Print and shaded views of the part. All mm, measured from the part's lowest x, y and z. Round coordinates to 2 decimals unless told otherwise and drop trailing zeros. Write each loop counter-clockwise with the first axis right and the second up, starting at its lowest first coordinate (ties: lowest second). Pieces come first, ordered by that corner, then holes. Notation, with made-up numbers: M 63,87.5 L 97,87.5 A7 ccw 97,92.5 Z; hole C 8.25,7 d6. An arc over 180 degrees is marked long. Write item = value, one per line.
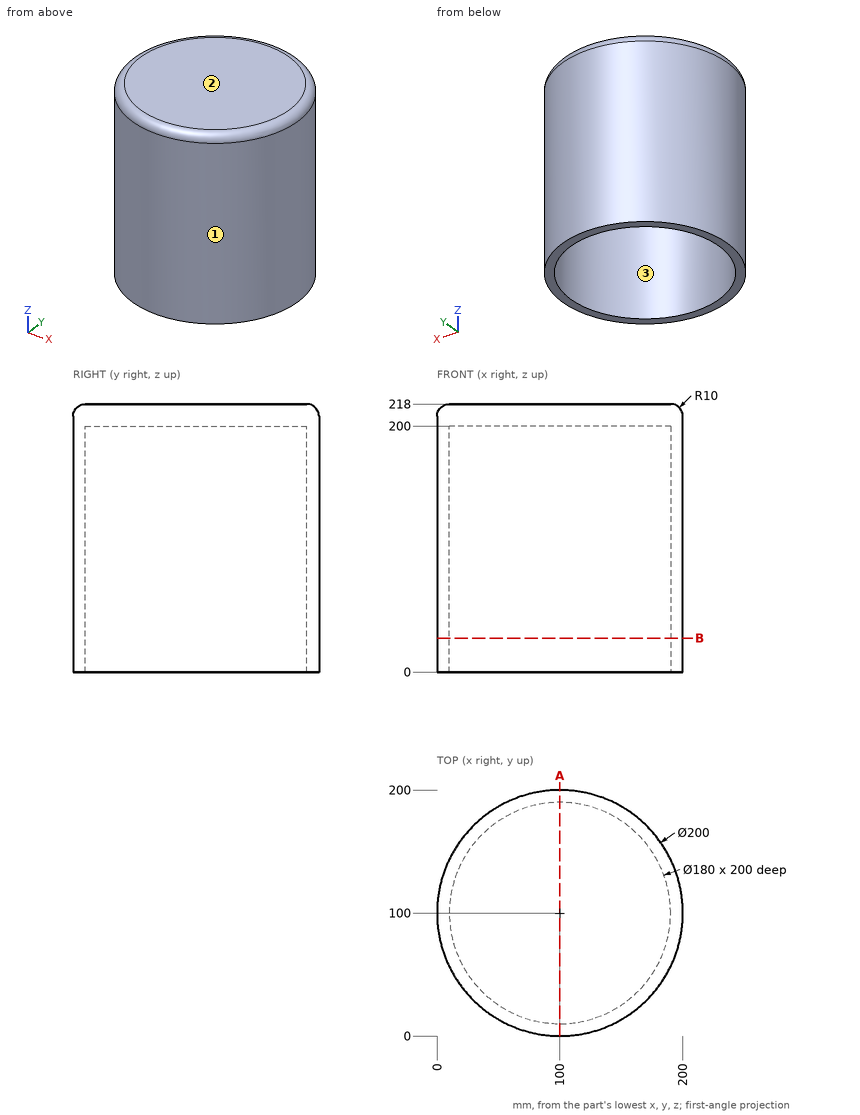
1. Mould opens along X. For the marked faces 1, 2 and 3 say: pulls with the +X half, pulls with the -X half, needs draft (parallel to the pull), parting line crosses it, or undercut.
Responses:
face_1 = parting line crosses it
face_2 = needs draft
face_3 = undercut
2. Band-saw the part on A-A (x = 100). List the corners of the cut face in (y, z).
Responses:
outline = M 0,0 L 10,0 L 10,200 L 190,200 L 190,0 L 200,0 L 200,208 A10 ccw 190,218 L 10,218 A10 ccw 0,208 Z
3. Flat gauge pins, fed straight in: pin 1 (2 mm diameter, centred on x = 126, y = 101.5, fed in from -Z); pin 2 (5 mm diameter, centred on x = 179.5, z = 79, fed in from +Y); pin 3 (8 mm diameter, centred on x = 67.5, z = 156, fed in from +Y). Where does each tip first touch, or does it go through?
Responses:
pin_1 = 200
pin_2 = 163.8
pin_3 = 195.85
4. Band-saw the part on B-B (z = 27.5). List the corners of the cut face in (x, y), plus the area to 3 significant figures.
Responses:
outline = C 100,100 d200; hole C 100,100 d180
area = 5,970 mm²
5. Probe probe 1 along Y at (x, z) = (100, 142); probe 2 along Z at (x, y) = (38, 62); probe 3 along Y at (x, z) = (22, 79). List the from-to ranges inside material, lowest first.
Responses:
probe_1 = 0 to 10, 190 to 200
probe_2 = 200 to 218
probe_3 = 37.42 to 55.1, 144.9 to 162.58
